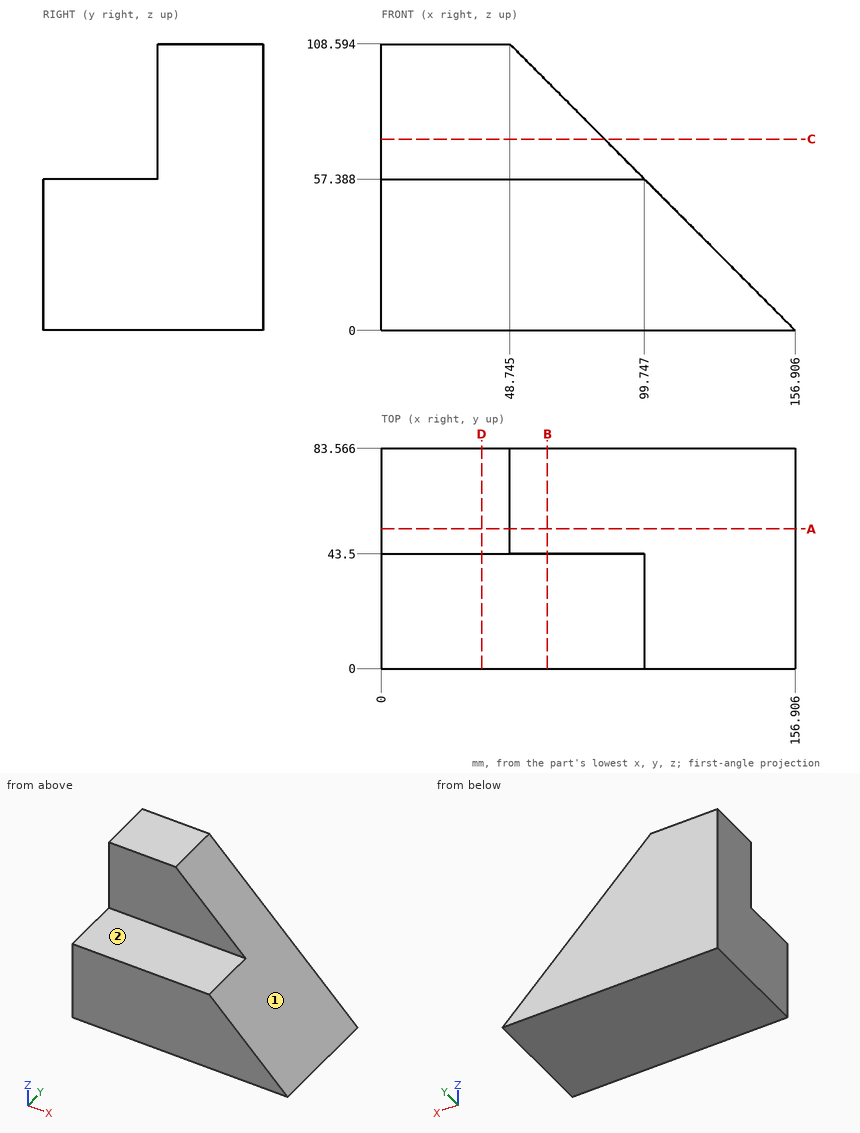
Geometry check sheet. Reference: drawing and pictorial views, mm from the part's lowest x, y, z. A direction names the side the tool comes from. Give positions to 0.01 mm unless a question says otherwise; leave off trailing zeros. Write each loop counter-clockwise with the first axis right and the second up, starting at its lowest first coordinate (ties: lowest second). Pieces come first, ordered by that corner, then holes. Notation, with made-up numbers: M -30,-39 L -26,-39 A21 cw -26,-19 Z; hole C 11.5,-1.75 d7. An arc over 180 degrees is marked long. Put each result on its own line as item: value. Start each with the question number.
1. Section check D-D (x = 38). Record the cut outline in (y, z), and give its area (3 significant figures).
2. Section check B-B (x = 63). Record the cut outline in (y, z), and give its area (3 significant figures).
3. Section check A-A (y = 53). Record the cut outline in (x, z) (1 decimal), and give its area (3 significant figures).
4. Scan lines: line 1 along Z through (x, y) = (41, 39.5); line 2 along Y through (x, z) = (44, 60.5); line 3 along X through (y, z) = (58.5, 103.5). Record each from-to range of solid material in increasing order. Write a range as [from, to].
5. Go/stop test with flat-tipped pins: pin 1 Ø4 at (x, z) = (70.5, 37) entering from -Y; pin 2 Ø10 at (y, z) = (45.5, 25.5) entering from +X; pin 3 Ø1 at (x, y) = (72.5, 65) entering from +Z (1 decimal); pin 4 Ø10 at (x, z) = (19.5, 67) entering from -Y. Record where each tip stops, or that it passes through.
6. Section check C-C (z = 72.5). Record the cut outline in (x, y) (1 decimal).
7. Set-up check for the marked faces 1 and 2: record each of +Z, -Z, +X, -X, +Y, -Y from which the full face is reachable in a straight line by a thin tool's end or side.
Answer list:
1. outline: M 0,0 L 83.57,0 L 83.57,108.59 L 43.5,108.59 L 43.5,57.39 L 0,57.39 Z
1. area: 6,850 mm2
2. outline: M 0,0 L 83.57,0 L 83.57,94.28 L 43.5,94.28 L 43.5,57.39 L 0,57.39 Z
2. area: 6,270 mm2
3. outline: M 0,0 L 156.9,0 L 48.7,108.6 L 0,108.6 Z
3. area: 11,200 mm2
4. line 1: [0, 57.39]
4. line 2: [43.5, 83.57]
4. line 3: [0, 53.82]
5. pin 1: y = 0
5. pin 2: x = 136.49
5. pin 3: z = 85.2
5. pin 4: y = 43.5
6. outline: M 0,43.5 L 84.7,43.5 L 84.7,83.6 L 0,83.6 Z
7. face 1: +Z, +X, +Y, -Y
7. face 2: +Z, +X, -X, -Y
